The model under review builds one solid part; all positions refer to its coordinate system, in mm. A direction names the side the tool comes from. Coordinates: 2 decimals unless noted, no trailing zeros. Write each loop counter-clockwise with the first axis right and the second up, starting at its lowest first coordinate (ties: lowest second). Pieces come first, ordered by that corner, then holes.
1) For line 1 (Y direction, x = -270, z = 0.35); line 2 (X direction, y = 139, z = 3.25); line 3 (X direction, y = 72.5, z = 3.55), list the stretches that pass through material, from the lowest coordinate up.
2) Add section A-A, the plane z = 1.1. Give the number of separate pieces and of enclosed holes in the cut face, then the cut area to 3 significant figures.
3) Add section C-C, the plane x = -153.5. State the section outline as (y, z) points, then the cut area to 3 significant figures.
4) Machinability: for faces 3 (the cylindrical face through (-139.774, 50.05, 2.465)), 4 (the cylindrical face through (-279.933, 32.609, 2.465)), 5 (the flat face through (-169, 58, 5)), which of the approach directions +Z, -Z, +X, -X, +Y, -Y give a long, thin tool a straight path to every point of the face, cutting with its end or side? Answer none if there is none.
5) For P1, Ø1.5, axis at x = -337.5, z = 2.5, coming from the +Y side; P2, Ø1.5, axis at y = 62.5, z = 2, coming from the +X side, all flat-tipped, find the tip position at first contact; note any pin that passes through.
6) Mouldability with a two-part tool opening along X and no side actions: class faces 1 (the flat face through (-169, 58, 0)), 2 (the cylindrical face through (-215.488, 40.585, 2.465)) as released by +X, released by -X, zero draft, split by the parting line, or undercut.
7) Add section B-B, the plane x = -93. State the section outline as (y, z) points.
from build123d import *

# Parameters (mm, degrees)
MODEL_R                  = 1.499999966
MODEL_W                  = 5.000000075
MODEL_H                  = 8.000000119
MODEL_W_2                = 5.000000074
MODEL_H_2                = 10.000000149
MODEL_H_3                = 8.00000012
MODEL_H_4                = 9.999934109
MODEL_W_3                = 10.000000149
MODEL_H_5                = 5.000000075
RESSALTO_EXTRUS_O1_DEPTH = 5


with BuildPart() as part:
    # Model → Ressalto-extrusão1 (new body)
    with BuildSketch(Plane.XY):
        with BuildLine():
            Line((8, -12), (-351.893274345, -12))
            ThreePointArc((-351.893274345, -12), (-354.083207051, -11.160599835), (-354.999940033, -9.001896861))
            Line((-354.999940033, -9.001896861), (-354.999940033, 156.005514216))
            ThreePointArc((-354.999940033, 156.005514216), (-354.121260376, 158.126834559), (-351.999940033, 159.005514216))
            Line((-351.999940033, 159.005514216), (-286.35488426, 159.005514216))
            ThreePointArc((-286.35488426, 159.005514216), (-284.233563917, 158.126834559), (-283.35488426, 156.005514216))
            Line((-283.35488426, 156.005514216), (-283.35488426, 109.0327131))
            ThreePointArc((-283.35488426, 109.0327131), (-282.183311385, 106.204285975), (-279.35488426, 105.0327131))
            Line((-279.35488426, 105.0327131), (-240.26491068, 105.0327131))
            Line((-240.26491068, 105.0327131), (-174.726717369, 105.0327131))
            Line((-174.726717369, 105.0327131), (-164.735516671, 105.0327131))
            ThreePointArc((-164.735516671, 105.0327131), (-161.199982765, 103.568247006), (-159.735516671, 100.0327131))
            Line((-159.735516671, 100.0327131), (-159.735516671, 99.000000432))
            ThreePointArc((-159.735516671, 99.000000432), (-139.232991354, 49.502525749), (-89.735516671, 29.000000432))
            Line((-89.735516671, 29.000000432), (-80.697953904, 29.000000432))
            ThreePointArc((-80.697953904, 29.000000432), (-40.9657847, 49.85268265), (-24.211685646, 91.479354272))
            Line((-24.211685646, 91.479354272), (-14.220289858, 91.479354272))
            Line((-14.220289858, 91.479354272), (-14.220289858, 96.379354272))
            Line((-14.220289858, 96.379354272), (-24.248305583, 96.379354272))
            ThreePointArc((-24.248305583, 96.379354272), (-37.455951456, 132.806572516), (-69.044817062, 155.245995598))
            ThreePointArc((-69.044817062, 155.245995598), (-72.433921946, 160.78421234), (-67.495803781, 165))
            Line((-67.495803781, 165), (8.006839019, 165))
            ThreePointArc((8.006839019, 165), (10.19856892, 164.048492138), (11, 161.797546694))
            Line((11, 161.797546694), (11, -9))
            ThreePointArc((11, -9), (10.121320344, -11.121320344), (8, -12))
        make_face()
        with Locations((-291.500004344, 51.500000767)):
            Circle(MODEL_R, mode=Mode.SUBTRACT)
        with Locations((-291.500004344, 138.500002064)):
            Circle(MODEL_R, mode=Mode.SUBTRACT)
        with Locations((-306.500004567, 138.500002064)):
            Circle(MODEL_R, mode=Mode.SUBTRACT)
        with Locations((-336.499940034, 51.48938817)):
            Circle(MODEL_R, mode=Mode.SUBTRACT)
        with Locations((-306.500004567, 51.500000767)):
            Circle(MODEL_R, mode=Mode.SUBTRACT)
        with Locations((-336.499992479, 138.499996904)):
            Circle(MODEL_R, mode=Mode.SUBTRACT)
        with Locations((-321.500004791, 138.500002064)):
            Circle(MODEL_R, mode=Mode.SUBTRACT)
        with Locations((-321.500004791, 51.500000767)):
            Circle(MODEL_R, mode=Mode.SUBTRACT)
        with Locations((-50.500000753, 15.500000231)):
            Circle(MODEL_R, mode=Mode.SUBTRACT)
        with Locations((-170.000002533, 95.000001416)):
            Circle(MODEL_R, mode=Mode.SUBTRACT)
        with Locations((-244.000003636, 95.000001416)):
            Circle(MODEL_R, mode=Mode.SUBTRACT)
        with Locations((-191.500002854, 15.500000231)):
            Circle(MODEL_R, mode=Mode.SUBTRACT)
        with Locations((-321.500004791, 42.000000626)):
            Rectangle(MODEL_W, MODEL_H, mode=Mode.SUBTRACT)
        with Locations((-321.499939997, 147.999896164)):
            Rectangle(MODEL_W_2, MODEL_H, mode=Mode.SUBTRACT)
        with Locations((-306.499940072, 147.999896164)):
            Rectangle(MODEL_W, MODEL_H, mode=Mode.SUBTRACT)
        with Locations((-336.500005014, 62.000000924)):
            Rectangle(MODEL_W_2, MODEL_H_2, mode=Mode.SUBTRACT)
        with Locations((-336.500005014, 42.000000626)):
            Rectangle(MODEL_W_2, MODEL_H, mode=Mode.SUBTRACT)
        with Locations((-321.500004791, 62.000000924)):
            Rectangle(MODEL_W, MODEL_H_2, mode=Mode.SUBTRACT)
        with Locations((-336.499939997, 147.999896164)):
            Rectangle(MODEL_W_2, MODEL_H, mode=Mode.SUBTRACT)
        with Locations((-306.500004567, 62.000000924)):
            Rectangle(MODEL_W_2, MODEL_H_2, mode=Mode.SUBTRACT)
        with Locations((-306.500004567, 42.000000626)):
            Rectangle(MODEL_W_2, MODEL_H, mode=Mode.SUBTRACT)
        with Locations((-321.499939997, 127.999958382)):
            Rectangle(MODEL_W_2, MODEL_H_2, mode=Mode.SUBTRACT)
        with Locations((-336.499939997, 127.999958382)):
            Rectangle(MODEL_W_2, MODEL_H_2, mode=Mode.SUBTRACT)
        with Locations((-306.499940072, 127.999958382)):
            Rectangle(MODEL_W, MODEL_H_2, mode=Mode.SUBTRACT)
        with Locations((-291.499939997, 147.999896164)):
            Rectangle(MODEL_W_2, MODEL_H, mode=Mode.SUBTRACT)
        with Locations((-291.499939997, 127.999958382)):
            Rectangle(MODEL_W_2, MODEL_H_2, mode=Mode.SUBTRACT)
        with Locations((-291.499939997, 41.999963457)):
            Rectangle(MODEL_W_2, MODEL_H_3, mode=Mode.SUBTRACT)
        with Locations((-291.499939997, 61.99993092)):
            Rectangle(MODEL_W_2, MODEL_H_4, mode=Mode.SUBTRACT)
        with BuildLine():
            Line((-283.35488426, 76.35164541), (-283.35488426, 41.000000433))
            ThreePointArc((-283.35488426, 41.000000433), (-279.840165634, 32.514719058), (-271.354884259, 29.000000432))
            Line((-271.354884259, 29.000000432), (-254.058912469, 29.000000432))
            ThreePointArc((-254.058912469, 29.000000432), (-215.005187795, 40.906914879), (-189.237444794, 72.576955029))
            ThreePointArc((-189.237444794, 72.576955029), (-190.205525947, 81.94100534), (-198.52230859, 86.35164541))
            Line((-198.52230859, 86.35164541), (-273.35488426, 86.35164541))
            ThreePointArc((-273.35488426, 86.35164541), (-280.425952072, 83.422713221), (-283.35488426, 76.35164541))
        make_face(mode=Mode.SUBTRACT)
        with Locations((-66.000000537, 15.500000038)):
            Rectangle(MODEL_W_3, MODEL_H_5, mode=Mode.SUBTRACT)
        with Locations((-35.004146846, 15.500000038)):
            Rectangle(MODEL_W_3, MODEL_H_5, mode=Mode.SUBTRACT)
        with Locations((-207.000000537, 15.500000038)):
            Rectangle(MODEL_W_3, MODEL_H_5, mode=Mode.SUBTRACT)
        with Locations((-176.004146697, 15.500000038)):
            Rectangle(MODEL_W_3, MODEL_H_5, mode=Mode.SUBTRACT)
    extrude(amount=RESSALTO_EXTRUS_O1_DEPTH)


solid = part.part
Geometry results:
1. line 1: y = -12 to 29, 86.35 to 105.03
1. line 2: x = -355 to -337.91, -335.09 to -322.91, -320.09 to -307.91, -305.09 to -292.91, -290.09 to -283.35, -42.82 to 11
1. line 3: x = -355 to -283.35, -189.27 to -154.53, -27.65 to 11
2. separate pieces: 1
2. enclosed holes: 33
2. area: 36,000 mm2
3. outline: (-12, 0) - (70.12, 0) - (70.12, 5) - (-12, 5) - close
3. area: 411 mm2
4. face 3: +Z, -Z, +Y
4. face 4: +Z, -Z
4. face 5: +Z, +X, -X, +Y, -Y
5. P1: stops at y = 159.01
5. P2: stops at x = 11
6. face 1: zero draft
6. face 2: undercut
7. outline: (-12, 0) - (29.08, 0) - (29.08, 5) - (-12, 5) - close
